Could you check a few things on this model? Use its own coordinates, in mm. A direction names the side the tool comes from. Coordinates: 2 decimals unless noted, no trailing zeros. Order: outer loops, then holes, each group sorted by start corner. A loop starts at its lowest first (then second) coordinate and runs counter-clockwise, first axis right, second up. Notation, with made-up numbers: M -24,34 L 14,34 A20 ccw 14,72 Z; hole C -3,31 d11. An arc over 180 degrees is marked long. One line per question, with ' | ' between items. Start each with the question number.
from build123d import *

# Parameters (mm, degrees)
F0_R     = 3
F0_R_2   = 12.7
F1_DEPTH = 12.7


# Not quite as in the source:
# - a feature names something its author has since deleted; it is built from what else it names


with BuildPart() as f1:
    # F0 (on Top) → F1 (new body)
    with BuildSketch(Plane.XY):
        with BuildLine():
            ThreePointArc((56.0618189529, -29.9999992666), (105.6598328516, -42.0377563289), (134.6028392714, 0))
            ThreePointArc((134.6028392714, 0), (105.6598328516, 42.0377563289), (56.0618189529, 29.9999992666))
            ThreePointArc((56.0618189529, 29.9999992666), (44.6028392714, 0), (56.0618189529, -29.9999992666))
        make_face()
        with Locations((89.6028392714, 0)):
            Circle(F0_R, mode=Mode.SUBTRACT)
        with BuildLine():
            ThreePointArc((84.5849392714, 8.08), (83.0886369502, 9.4747414442), (84.3749411096, 11.0652275152))
            ThreePointArc((84.3749411096, 11.0652275152), (84.5827763317, 11.0799984406), (84.7906532876, 11.0658269561))
            Line((84.7906532876, 11.0658269561), (94.6185763317, 11.0799984406))
            ThreePointArc((94.6185763317, 11.0799984406), (95.6806344526, 10.641424611), (96.1207392714, 9.58))
            ThreePointArc((96.1207392714, 9.58), (95.6813994432, 8.5193398282), (94.6207392714, 8.08))
            Line((94.6207392714, 8.08), (84.5849392714, 8.08))
        make_face(mode=Mode.SUBTRACT)
        with BuildLine():
            ThreePointArc((56.0618189529, -29.9999992666), (44.6028392714, 0), (56.0618189529, 29.9999992666))
            Line((56.0618189529, 29.9999992666), (0, 29.9999992666))
            ThreePointArc((0, 29.9999992666), (8.4967360104, 16.0569935802), (11.4589796815, 0))
            ThreePointArc((11.4589796815, 0), (8.4967360104, -16.0569935802), (0, -29.9999992666))
            Line((0, -29.9999992666), (56.0618189529, -29.9999992666))
        make_face()
        with BuildLine():
            ThreePointArc((11.4589796815, 0), (8.4967360104, 16.0569935802), (0, 29.9999992666))
            ThreePointArc((0, 29.9999992666), (-78.5410203185, 0), (0, -29.9999992666))
            ThreePointArc((0, -29.9999992666), (8.4967360104, -16.0569935802), (11.4589796815, 0))
        make_face()
        with Locations((-33.5410203185, 0)):
            Circle(F0_R_2, mode=Mode.SUBTRACT)
    extrude(amount=F1_DEPTH)


solid = f1.part
(1) Imagine slicing it at B-B, the plane z = 2.5. Write out the boundary of the cut face in (x, y), plus the area to 3 significant figures.
(2) Imagine slicing it at D-D, the plane y = 39.5. Write out the boundary of the cut face in (x, z).
(3) We'd pull the mould along X, two halves only. Please class faces 1 (the cylindrical face through (134.577, -1.519, 6.261)), 2 (the flat face through (27, 1, 0)), 3 (the cylindrical face through (92.464, 0.901, 6.261)): +X half, -X half, draft (parallel to the pull), parting line (faces both ways), or undercut.
(4) Imagine slicing it at A-A, the plane y = 0. Write out the boundary of the cut face in (x, z).
(5) On a 3-axis mill with a long thin cutter (end or side, diameter ignored), from which of +Z, -Z, +X, -X, +Y, -Y can I reach the whole of each face in a straight line? I mean faces 4 (the flat face through (90, 8.08, 6)), 5 (the flat face through (28, -30, 6)), 6 (the flat face through (28, 30, 6)). Say none if no direction works.
(6) If I drill on line 1 along X through (y, z) = (-1, 6); line 2 along Y through (x, z) = (-42, 2.75); line 3 along Y through (x, z) = (22, 9), over which ranges is the centre line in solid material (lowest first)? Write a range as from..to.
(7) Imagine slicing it at C-C, the plane x = -37. Write out the boundary of the cut face in (y, z), plus the area to 3 significant figures.
(8) For P1, Ø3, axis at x = 88, z = 3, coming from the +Y side; P2, Ø4, axis at x = 21, z = 5, coming from the +Y side; P3, Ø1, axis at y = -12.5, z = 4.5, coming from the +X side; P4, Ø1.5, axis at y = -19.5, z = 8, coming from the -X side, each with a flat end and sliding along its axis, tell me the tip position at first contact or that it passes through.
Answers:
1) outline: M 0,-30 L 56.06,-30 A45 ccw long 56.06,30 L 0,30 A45 ccw long Z; hole C -33.54,0 d25.4; hole M 84.58,8.08 L 94.62,8.08 A1.5 ccw 94.62,11.08 L 84.79,11.07 A1.5 ccw long Z; hole C 89.6,0 d6 | area: 14,600 mm²
2) outline: M -55.1,0 L -11.98,0 L -11.98,12.7 L -55.1,12.7 Z; M 68.04,0 L 111.16,0 L 111.16,12.7 L 68.04,12.7 Z
3) face 1: undercut | face 2: draft | face 3: undercut
4) outline: M -78.54,0 L -46.24,0 L -46.24,12.7 L -78.54,12.7 Z; M -20.84,0 L 86.6,0 L 86.6,12.7 L -20.84,12.7 Z; M 92.6,0 L 134.6,0 L 134.6,12.7 L 92.6,12.7 Z
5) face 4: +Z, -Z | face 5: +Z, -Z, -Y | face 6: +Z, -Z, +Y
6) line 1: -78.53..-46.2, -20.88..86.77, 92.43..134.59 | line 2: -44.2..-9.47, 9.47..44.2 | line 3: -30..30
7) outline: M -44.87,0 L -12.22,0 L -12.22,12.7 L -44.87,12.7 Z; M 12.22,0 L 44.87,0 L 44.87,12.7 L 12.22,12.7 Z | area: 829 mm²
8) P1: y = 45 | P2: y = 30 | P3: x = 132.97 | P4: x = -74.45
